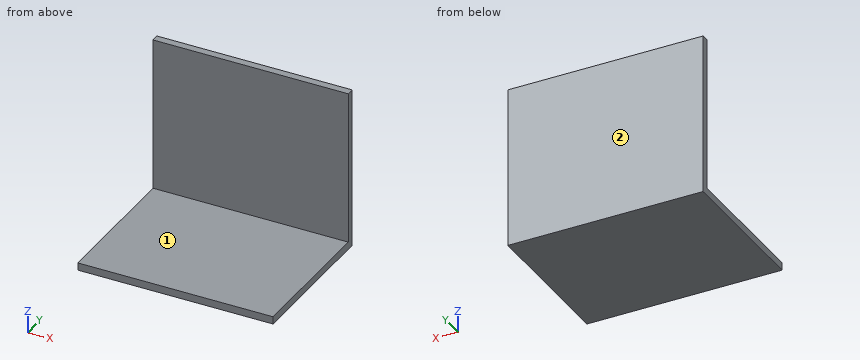
```python
from build123d import *

# Parameters (mm, degrees)
ESQUISSE1_W             = 52
ESQUISSE1_H             = 40
BOSS_EXTRU_1_DEPTH      = 43
ESQUISSE2_W             = 48.222048012
ESQUISSE2_H             = 36
ENL_V_MAT_EXTRU_1_DEPTH = 50
ESQUISSE3_W             = 72.686110251
ESQUISSE3_H             = 50.534375484
ENL_V_MAT_EXTRU_2_DEPTH = 38


with BuildPart() as part:
    # Esquisse1 → Boss.-Extru.1 (new body)
    with BuildSketch(Plane.XY):
        Rectangle(ESQUISSE1_W, ESQUISSE1_H)
    extrude(amount=BOSS_EXTRU_1_DEPTH)

    # Esquisse2 → Enlèv. mat.-Extru.1 (cut)
    with BuildSketch(Plane.ZY.offset(26)):
        with Locations((26.111024006, 0)):
            Rectangle(ESQUISSE2_W, ESQUISSE2_H)
    extrude(amount=-ENL_V_MAT_EXTRU_1_DEPTH, mode=Mode.SUBTRACT)

    # Esquisse3 → Enlèv. mat.-Extru.2 (cut)
    with BuildSketch(Plane.XZ.offset(20)):
        with Locations((1.657877156, 27.267187742)):
            Rectangle(ESQUISSE3_W, ESQUISSE3_H)
    extrude(amount=-ENL_V_MAT_EXTRU_2_DEPTH, mode=Mode.SUBTRACT)


solid = part.part
```
Could you check a few things on this model? Use its own coordinates, in mm. Face numbers are marked on the shaded views. A direction names the side the tool comes from. Round coordinates to 2 decimals unless told otherwise and drop trailing zeros. Write each loop counter-clockwise with the first axis right and the second up, starting at its lowest first coordinate (ties: lowest second). Pieces come first, ordered by that corner, then holes. Notation, with made-up numbers: M 39.25,3.5 L 52.25,3.5 A17 cw 52.25,23.5 Z; hole C 50,29.25 d7. An arc over 180 degrees is marked long. Answer in a Markdown table with one row per item. Add a question column.
Q1. Will these pins go through, and if not, where does the flat tip stop? pin 1 Ø12 at (x, z) = (19.5, 34.5) entering from -Y; pin 2 Ø1.5 at (x, y) = (2.5, -4.5) entering from +Z.
Q2. Imagine slicing it at C-C (y = -8.5). Please give me the cut outline in (x, z), then the cut area to 3 significant figures.
Q3. On a 3-axis mill with a long thin cutter (end or side, diameter ignored), from which of +Z, -Z, +X, -X, +Y, -Y can I reach the whole of each face in a straight line? I mean the marked faces 1 and 2. Say none if no direction works.
Q4. If I drill on line 1 (Y direction, x = -23.5, z = 25.5); line 2 (Z direction, x = -18, y = 17.5), over which ranges is the centre line in solid material (lowest first)? Write a range as from..to.
Q5. Imagine slicing it at A-A (x = 8). Please give me the cut outline in (y, z), then the cut area to 3 significant figures.
Q6. Imagine slicing it at B-B (z = 17). Please give me the cut outline in (x, y).
Values:
| question | item | result |
|---|---|---|
| 1 | pin 1 | y = 18 |
| 1 | pin 2 | z = 2 |
| 2 | outline | M -26,0 L 26,0 L 26,2 L -26,2 Z |
| 2 | area | 104 mm^2 |
| 3 | face 1 | +Z, +X, -X, -Y |
| 3 | face 2 | +Z, -Z, +X, -X, +Y |
| 4 | line 1 | 18..20 |
| 4 | line 2 | 0..2 |
| 5 | outline | M -20,0 L 20,0 L 20,43 L 18,43 L 18,2 L -20,2 Z |
| 5 | area | 162 mm^2 |
| 6 | outline | M -26,18 L 26,18 L 26,20 L -26,20 Z |
